```python
from build123d import *

# Parameters (mm, degrees)
BOSS_EXTRUDE1_DEPTH        = 11.938
F_4_5_4_5_DIAMETER_HOLE1_D = 4.5
CUT_EXTRUDE1_DEPTH         = 2.54


with BuildPart() as part:
    # Sketch1 → Boss-Extrude1 (new body)
    with BuildSketch(Plane(origin=(0, 0, 0), x_dir=(1, 0, 0), z_dir=(0, 1, 0))):
        with BuildLine():
            Line((0, 9.525), (190.5, 9.525))
            ThreePointArc((190.5, 9.525), (200.025, 0), (190.5, -9.525))
            Line((190.5, -9.525), (0, -9.525))
            ThreePointArc((0, -9.525), (-9.525, 0), (0, 9.525))
        make_face()
    extrude(amount=BOSS_EXTRUDE1_DEPTH)

    # Ø4.5 (4.5) Diameter Hole1 (through all)
    with Locations(Plane(origin=(0, 11.938, 0), x_dir=(1, 0, 0), z_dir=(0, 1, 0))):
        with Locations((0, 0)):
            Hole(F_4_5_4_5_DIAMETER_HOLE1_D / 2)

    # Sketch5 → Cut-Extrude1 (cut)
    with BuildSketch(Plane.XZ):
        with BuildLine():
            Line((10.972725624, 9.525), (0, 9.525))
            ThreePointArc((0, 9.525), (-9.525, 0), (0, -9.525))
            Line((0, -9.525), (10.972725624, -9.525))
            Line((10.972725624, -9.525), (10.972725624, -6.985))
            Line((10.972725624, -6.985), (11.934096284, -4.34365582))
            ThreePointArc((11.934096284, -4.34365582), (12.7, 0), (11.934096284, 4.34365582))
            Line((11.934096284, 4.34365582), (10.972725624, 6.985))
            Line((10.972725624, 6.985), (10.972725624, 9.525))
        make_face()
    extrude(amount=-CUT_EXTRUDE1_DEPTH, mode=Mode.SUBTRACT)


solid = part.part
```
Verification items for the finished model (mm, model axes). Round coordinates to 2 decimals unless told otherwise and drop trailing zeros. Write each loop counter-clockwise with the first axis right and the second up, starting at its lowest first coordinate (ties: lowest second). Pieces come first, ordered by that corner, then holes.
1. Section check B-B on y = 6.75. Enter the section's corners in (x, z) (3 decimals).
2. Scan lines: L1, parallel to X at y = 9.25, z = -0.25; L2, parallel to X at y = 9.25, z = 1.25; L3, parallel to Y at x = 4.5, z = 6.25. Record each from-to range of solid material in increasing order.
3. Gauge pin test, flat end, axial feed: P1, Ø2, axis at y = 1, z = -8, coming from the -X side. Record the tip position at first contact, or that the pin passes through.
4. Draft check along X on faces 1 (the flat face through (107, 0, 0)), 2 (the cylindrical face through (-9.523, 7.173, 0.209)), 3 (the cylindrical face through (0.29, 7.17, -2.23)). Enter one of: +X half, -X half, draft (parallel to the pull), parting line (faces both ways), or undercut.
5. Section check A-A on z = 0. Enter the section's corners in (x, y) (3 decimals), plus the area to 3 significant figures.
Answer:
1. outline: (0, -9.525) - (190.5, -9.525) arc R9.525 ccw to (190.5, 9.525) - (0, 9.525) arc R9.525 ccw to start; hole circle Ø4.5 at (0, 0)
2. L1: x = -9.52 to -2.24, 2.24 to 200.02
2. L2: x = -9.44 to -1.87, 1.87 to 199.94
2. L3: y = 2.54 to 11.94
3. P1: stops at x = 10.97
4. face 1: draft
4. face 2: -X half
4. face 3: undercut
5. outline: (-9.525, 2.54) - (-2.25, 2.54) - (-2.25, 11.938) - (-9.525, 11.938) - close; (2.25, 2.54) - (12.7, 2.54) - (12.7, 0) - (200.025, 0) - (200.025, 11.938) - (2.25, 11.938) - close
5. area: 2,400 mm2
